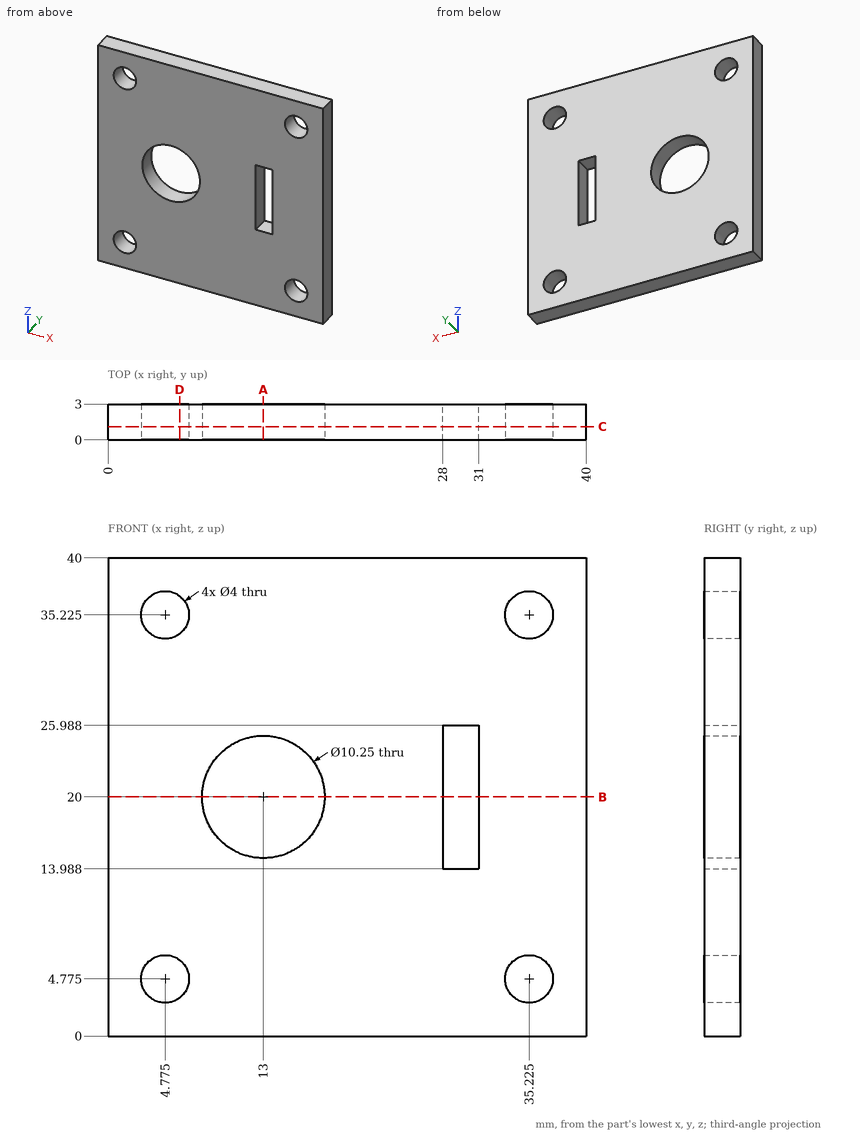
Answer from the drawing. Dimensions are ordinates in mm from the lowest x, y and z of the part. Coordinates: 2 decimals unless noted, no trailing zeros. Loops run counter-clockwise (first coordinate to the right, second up) from the corner with the lowest first, then second, coordinate; pieces in that order, holes last. Notation, with made-up numbers: (16.5, 11) -> (75.5, 11) arc R21 ccw to (75.5, 44) -> close; hole circle Ø7 at (-0.5, 86). An arc over 180 degrees is marked (long way). Answer as CSV lines item,"result".
Q1. Find the intervals of material crossed by probe 1 along Z at (x, y) = (29, 1.3); probe 2 along X at (y, z) = (0.15, 16) (1 decimal); probe 3 along Z at (x, y) = (4, 2.3), in increasing order.
Findings:
probe 1,"z = 0 to 13.99, 25.99 to 40"
probe 2,"x = 0 to 9.8, 16.2 to 28, 31 to 40"
probe 3,"z = 0 to 2.93, 6.62 to 33.38, 37.07 to 40"
Q2. The part is cut by section A-A on x = 13. Write down the section's boundary in (y, z) (1 decimal).
Findings:
outline,"(0, 0) -> (3, 0) -> (3, 14.9) -> (0, 14.9) -> close; (0, 25.1) -> (3, 25.1) -> (3, 40) -> (0, 40) -> close"
Q3. The part is cut by section C-C on y = 1.1. State how many separate pieces and enclosed holes the cut face has, and give its area (3 significant figures).
Findings:
separate pieces,"1"
enclosed holes,"6"
area,"1,430 mm²"
Q4. The part is cut by section B-B on z = 20. Write down the section's boundary in (x, y) (1 decimal).
Findings:
outline,"(0, 0) -> (7.9, 0) -> (7.9, 3) -> (0, 3) -> close; (18.1, 0) -> (28, 0) -> (28, 3) -> (18.1, 3) -> close; (31, 0) -> (40, 0) -> (40, 3) -> (31, 3) -> close"
Q5. The part is cut by section D-D on x = 6. Write down the section's boundary in (y, z), and give its area (3 significant figures).
Findings:
outline,"(0, 0) -> (3, 0) -> (3, 3.19) -> (0, 3.19) -> close; (0, 6.36) -> (3, 6.36) -> (3, 33.64) -> (0, 33.64) -> close; (0, 36.81) -> (3, 36.81) -> (3, 40) -> (0, 40) -> close"
area,"101 mm²"
